Input: part model. Units: mm. Frame: model coordinates. A direction names the side the tool comes from. Coordinates: 2 decimals unless noted, no trailing zeros. Loops run counter-clockwise (first coordinate to the right, second up) from the corner with the lowest first, then second, coordinate; pieces in that order, holes last.
Item 1: Section D-D on z = -22.5. Return loops of the section in (x, y).
Item 2: Ray query, line 1 along X through (y, z) = (45.9, 2.9) (3 decimals); line 2 along Y through (x, z) = (-42.6, 3.95) (3 decimals); line 3 along Y through (x, z) = (59, 1.35) (3 decimals). Return the intervals inside material, ascending.
Item 3: Section C-C on x = -42.6. Return loops of the section in (y, z) (3 decimals), and give its area (3 significant figures).
Item 4: Contact query for flat-ended pins moving along their axis: P1, Ø8.5, axis at x = -42.6, y = 45.9, coming from the -Z side; P2, Ø5.5, axis at x = 8.2, y = -56.4, coming from the +Z side; P3, Ø6, axis at x = -43.5, z = -10.5, coming from the +Y side; P4, Ø3, axis at x = -50, z = -4.5, coming from the +Y side. Output: stop coordinate, or through.
Item 5: Reachability of faces 4 (the flat face through (-1, 3, 0)), 5 (the cylindrical face through (62.03, 46.85, 2.85)) from +Z, -Z, +X, -X, +Y, -Y: full face, straight path, thin tool, end or side. Return the list, or none.
Item 6: Section A-A on x = 77. Return loops of the section in (y, z).
Item 7: Section B-B on y = 45.9. Return loops of the section in (x, z) (3 decimals), and give its area (3 significant figures).
Item 8: Pull-direction query (Y, two-part tool) for faces 1 (the cylindrical face through (5.68, -58.33, 2.85)), 2 (the flat face through (1, -73.66, -7)), 3 (the flat face through (79, -77, -40.64)); classes: released by +Y, released by -Y, zero draft, split by the parting line, or undercut.
```python
from build123d import *

# Parameters (mm, degrees)
SKETCH1_W                  = 169
SKETCH1_H                  = 152.4
BOSS_EXTRUDE1_DEPTH        = 2.54
SKETCH2_W                  = 169
SKETCH2_H                  = 2.54
BOSS_EXTRUDE2_DEPTH        = 40.64
CUT_EXTRUDE1_REACH         = 122.823
SKETCH4_R                  = 3.175
CUT_EXTRUDE2_REACH         = 178.776
SKETCH3_R                  = 3.020871564
SKETCH3_R_2                = 97.5
CONVERT_SOLID1_START       = -5.790000104
CONVERT_SOLID1_OUTLINE_W   = 169
CONVERT_SOLID1_OUTLINE_H   = 149.86
CONVERT_SOLID1_OUTLINE_R   = 3.175
CONVERT_SOLID1_DEPTH       = 11.580006304
CONVERT_SOLID1_START_2     = -40.64
CONVERT_SOLID1_2_OUTLINE_W = 169
CONVERT_SOLID1_2_OUTLINE_H = 3.2500062
CONVERT_SOLID1_2_DEPTH     = 43.18
CONVERT_SOLID1_START_3     = 2.54
CONVERT_SOLID1_3_OUTLINE_W = 169
CONVERT_SOLID1_3_OUTLINE_H = 2.54
CONVERT_SOLID1_3_DEPTH     = 2.060276352
CONVERT_SOLID1_START_4     = -67.869999896
CONVERT_SOLID1_4_OUTLINE_W = 169
CONVERT_SOLID1_4_OUTLINE_H = 5.790000104
CONVERT_SOLID1_4_DEPTH     = 144.069999896
CONVERT_SOLID1_START_5     = -79.4500062
CONVERT_SOLID1_5_OUTLINE_R = 3.020871564
CONVERT_SOLID1_5_DEPTH     = 3.2500062
CONVERT_SOLID1_6_OUTLINE_W = 169
CONVERT_SOLID1_6_OUTLINE_H = 2.54
CONVERT_SOLID1_6_DEPTH     = 0.546460785
CONVERT_SOLID1_START_6     = -85
CONVERT_SOLID1_7_DEPTH     = 170


with BuildPart() as part:
    # Sketch1 → Boss-Extrude1 (new body)
    with BuildSketch(Plane.XY):
        Rectangle(SKETCH1_W, SKETCH1_H)
    extrude(amount=BOSS_EXTRUDE1_DEPTH)

    # Sketch2 → Boss-Extrude2 (add)
    with BuildSketch(Plane(origin=(0, 0, 0), x_dir=(-1, 0, 0), z_dir=(0, 0, -1))):
        with Locations((0, -74.93)):
            Rectangle(SKETCH2_W, SKETCH2_H)
    extrude(amount=BOSS_EXTRUDE2_DEPTH)

    # Sketch4 → Cut-Extrude1 (cut, up to next)
    with BuildSketch(Plane(origin=(0, 0, 0), x_dir=(-1, 0, 0), z_dir=(0, 0, -1)), mode=Mode.PRIVATE) as cut_extrude1_sk1:
        with Locations((-59, 45.9)):
            Circle(SKETCH4_R)
    cut_extrude1_tool1 = extrude(cut_extrude1_sk1.sketch, amount=-CUT_EXTRUDE1_REACH, mode=Mode.PRIVATE) & part.part
    # Sketch4 → Cut-Extrude1 (cut, up to next)
    with BuildSketch(Plane(origin=(0, 0, 0), x_dir=(-1, 0, 0), z_dir=(0, 0, -1)), mode=Mode.PRIVATE) as cut_extrude1_sk2:
        with Locations((-59, -56.4)):
            Circle(SKETCH4_R)
    cut_extrude1_tool2 = extrude(cut_extrude1_sk2.sketch, amount=-CUT_EXTRUDE1_REACH, mode=Mode.PRIVATE) & part.part
    # Sketch4 → Cut-Extrude1 (cut, up to next)
    with BuildSketch(Plane(origin=(0, 0, 0), x_dir=(-1, 0, 0), z_dir=(0, 0, -1)), mode=Mode.PRIVATE) as cut_extrude1_sk3:
        with Locations((-8.2, 45.9)):
            Circle(SKETCH4_R)
    cut_extrude1_tool3 = extrude(cut_extrude1_sk3.sketch, amount=-CUT_EXTRUDE1_REACH, mode=Mode.PRIVATE) & part.part
    # Sketch4 → Cut-Extrude1 (cut, up to next)
    with BuildSketch(Plane(origin=(0, 0, 0), x_dir=(-1, 0, 0), z_dir=(0, 0, -1)), mode=Mode.PRIVATE) as cut_extrude1_sk4:
        with Locations((42.6, 45.9)):
            Circle(SKETCH4_R)
    cut_extrude1_tool4 = extrude(cut_extrude1_sk4.sketch, amount=-CUT_EXTRUDE1_REACH, mode=Mode.PRIVATE) & part.part
    # Sketch4 → Cut-Extrude1 (cut, up to next)
    with BuildSketch(Plane(origin=(0, 0, 0), x_dir=(-1, 0, 0), z_dir=(0, 0, -1)), mode=Mode.PRIVATE) as cut_extrude1_sk5:
        with Locations((42.6, -56.4)):
            Circle(SKETCH4_R)
    cut_extrude1_tool5 = extrude(cut_extrude1_sk5.sketch, amount=-CUT_EXTRUDE1_REACH, mode=Mode.PRIVATE) & part.part
    # Sketch4 → Cut-Extrude1 (cut, up to next)
    with BuildSketch(Plane(origin=(0, 0, 0), x_dir=(-1, 0, 0), z_dir=(0, 0, -1)), mode=Mode.PRIVATE) as cut_extrude1_sk6:
        with Locations((-8.2, -56.4)):
            Circle(SKETCH4_R)
    cut_extrude1_tool6 = extrude(cut_extrude1_sk6.sketch, amount=-CUT_EXTRUDE1_REACH, mode=Mode.PRIVATE) & part.part
    add(cut_extrude1_tool1.solids().sort_by_distance((59, 45.9, 0))[0], mode=Mode.SUBTRACT)
    add(cut_extrude1_tool2.solids().sort_by_distance((59, -56.4, 0))[0], mode=Mode.SUBTRACT)
    add(cut_extrude1_tool3.solids().sort_by_distance((8.2, 45.9, 0))[0], mode=Mode.SUBTRACT)
    add(cut_extrude1_tool4.solids().sort_by_distance((-42.6, 45.9, 0))[0], mode=Mode.SUBTRACT)
    add(cut_extrude1_tool5.solids().sort_by_distance((-42.6, -56.4, 0))[0], mode=Mode.SUBTRACT)
    add(cut_extrude1_tool6.solids().sort_by_distance((8.2, -56.4, 0))[0], mode=Mode.SUBTRACT)

    # Sketch3 → Cut-Extrude2 (cut, up to next)
    with BuildSketch(Plane(origin=(0, -73.66, 0), x_dir=(1, 0, 0), z_dir=(0, 1, 0)), mode=Mode.PRIVATE) as cut_extrude2_sk1:
        with Locations(Location((77, 28.473587136, 0), (0, 0, 180))):
            Circle(SKETCH3_R)
    cut_extrude2_tool1 = extrude(cut_extrude2_sk1.sketch, amount=-CUT_EXTRUDE2_REACH, mode=Mode.PRIVATE) & part.part
    # Sketch3 → Cut-Extrude2 (cut, up to next)
    with BuildSketch(Plane(origin=(0, -73.66, 0), x_dir=(1, 0, 0), z_dir=(0, 1, 0)), mode=Mode.PRIVATE) as cut_extrude2_sk2:
        with Locations(Location((-77, 28.473587136, 0), (0, 0, 180))):
            Circle(SKETCH3_R)
    cut_extrude2_tool2 = extrude(cut_extrude2_sk2.sketch, amount=-CUT_EXTRUDE2_REACH, mode=Mode.PRIVATE) & part.part
    # Sketch3 → Cut-Extrude2 (cut, up to next)
    with BuildSketch(Plane(origin=(0, -73.66, 0), x_dir=(1, 0, 0), z_dir=(0, 1, 0)), mode=Mode.PRIVATE) as cut_extrude2_sk3:
        with Locations((0, 105.473587136)):
            Circle(SKETCH3_R_2)
    cut_extrude2_tool3 = extrude(cut_extrude2_sk3.sketch, amount=-CUT_EXTRUDE2_REACH, mode=Mode.PRIVATE) & part.part
    add(cut_extrude2_tool1.solids().sort_by_distance((77, -73.66, -28.473587))[0], mode=Mode.SUBTRACT)
    add(cut_extrude2_tool2.solids().sort_by_distance((-77, -73.66, -28.473587))[0], mode=Mode.SUBTRACT)
    add(cut_extrude2_tool3.solids().sort_by_distance((0, -73.66, -105.473587))[0], mode=Mode.SUBTRACT)

    # Convert-Solid1: read off the stored shape, not the designer's step
    # Convert-Solid1 outline → Convert-Solid1 (add)
    with BuildSketch(Plane.XY.offset(CONVERT_SOLID1_START)):
        with Locations((0, 1.27)):
            Rectangle(CONVERT_SOLID1_OUTLINE_W, CONVERT_SOLID1_OUTLINE_H)
        with Locations((-42.6, -56.4)):
            Circle(CONVERT_SOLID1_OUTLINE_R, mode=Mode.SUBTRACT)
        with Locations((8.2, -56.4)):
            Circle(CONVERT_SOLID1_OUTLINE_R, mode=Mode.SUBTRACT)
        with Locations((59, -56.4)):
            Circle(CONVERT_SOLID1_OUTLINE_R, mode=Mode.SUBTRACT)
        with Locations((-42.6, 45.9)):
            Circle(CONVERT_SOLID1_OUTLINE_R, mode=Mode.SUBTRACT)
        with Locations((8.2, 45.9)):
            Circle(CONVERT_SOLID1_OUTLINE_R, mode=Mode.SUBTRACT)
        with Locations((59, 45.9)):
            Circle(CONVERT_SOLID1_OUTLINE_R, mode=Mode.SUBTRACT)
    extrude(amount=CONVERT_SOLID1_DEPTH)

    # Convert-Solid1 2 outline → Convert-Solid1 2 (add)
    with BuildSketch(Plane.XY.offset(CONVERT_SOLID1_START_2)):
        with Locations((0, -77.8250031)):
            Rectangle(CONVERT_SOLID1_2_OUTLINE_W, CONVERT_SOLID1_2_OUTLINE_H)
    extrude(amount=CONVERT_SOLID1_2_DEPTH)

    # Convert-Solid1 3 outline → Convert-Solid1 3 (add)
    with BuildSketch(Plane.XY.offset(CONVERT_SOLID1_START_3)):
        with Locations((0, -74.93)):
            Rectangle(CONVERT_SOLID1_3_OUTLINE_W, CONVERT_SOLID1_3_OUTLINE_H)
    extrude(amount=CONVERT_SOLID1_3_DEPTH)

    # Convert-Solid1 4 outline → Convert-Solid1 4 (cut)
    with BuildSketch(Plane(origin=(0, 0, 0), x_dir=(1, 0, 0), z_dir=(0, 1, 0)).offset(CONVERT_SOLID1_START_4)):
        with Locations((0, 2.895000052)):
            Rectangle(CONVERT_SOLID1_4_OUTLINE_W, CONVERT_SOLID1_4_OUTLINE_H)
    extrude(amount=CONVERT_SOLID1_4_DEPTH, mode=Mode.SUBTRACT)

    # Convert-Solid1 5 outline → Convert-Solid1 5 (cut)
    with BuildSketch(Plane(origin=(0, 0, 0), x_dir=(1, 0, 0), z_dir=(0, 1, 0)).offset(CONVERT_SOLID1_START_5)):
        with BuildLine():
            Line((72.820711196, 40.64), (-72.820711196, 40.64))
            ThreePointArc((-72.820711196, 40.64), (0, 7.973587136), (72.820711196, 40.64))
        make_face()
        with Locations((-77, 28.473587136)):
            Circle(CONVERT_SOLID1_5_OUTLINE_R)
        with Locations((77, 28.473587136)):
            Circle(CONVERT_SOLID1_5_OUTLINE_R)
    extrude(amount=CONVERT_SOLID1_5_DEPTH, mode=Mode.SUBTRACT)

    # Convert-Solid1 6 outline → Convert-Solid1 6 (cut)
    with BuildSketch(Plane(origin=(0, 0, 0), x_dir=(1, 0, 0), z_dir=(0, 1, 0)).offset(CONVERT_SOLID1_START_5)):
        with Locations((0, -1.27)):
            Rectangle(CONVERT_SOLID1_6_OUTLINE_W, CONVERT_SOLID1_6_OUTLINE_H)
    extrude(amount=CONVERT_SOLID1_6_DEPTH, mode=Mode.SUBTRACT)

    # Convert-Solid1 7 outline → Convert-Solid1 7 (cut)
    with BuildSketch(Plane.YZ.offset(CONVERT_SOLID1_START_6)):
        with BuildLine():
            Line((-67.869999896, -5.790000104), (-67.869999896, 0))
            ThreePointArc((-67.869999896, 0), (-71.964148233, -1.695851767), (-73.66, -5.790000104))
            Line((-73.66, -5.790000104), (-67.869999896, -5.790000104))
        make_face()
        with BuildLine():
            ThreePointArc((-79.4500062, -5.790000104), (-76.05830088, 2.39830088), (-67.869999896, 5.7900062))
            Line((-67.869999896, 5.7900062), (-73.66, 5.7900062))
            Line((-73.66, 5.7900062), (-73.66, 4.600276352))
            Line((-73.66, 4.600276352), (-76.2, 4.600276352))
            Line((-76.2, 4.600276352), (-76.2, 2.54))
            Line((-76.2, 2.54), (-78.903545415, 2.54))
            Line((-78.903545415, 2.54), (-78.903545415, 0))
            Line((-78.903545415, 0), (-79.4500062, 0))
            Line((-79.4500062, 0), (-79.4500062, -5.790000104))
        make_face()
    extrude(amount=CONVERT_SOLID1_7_DEPTH, mode=Mode.SUBTRACT)


solid = part.part
```
Results found:
1. outline: (-84.5, -79.45) - (-51.2, -79.45) - (-51.2, -73.66) - (-84.5, -73.66) - close; (51.2, -79.45) - (84.5, -79.45) - (84.5, -73.66) - (51.2, -73.66) - close
2. line 1: x = -84.5 to -45.775, -39.425 to 5.025, 11.375 to 55.825, 62.175 to 84.5
2. line 2: y = -74.133 to -59.575, -53.225 to 42.725, 49.075 to 76.2
2. line 3: y = -76.987 to -59.575, -53.225 to 42.725, 49.075 to 76.2
3. outline: (-79.45, -17.772) - (-73.66, -17.772) - (-73.66, -5.79) arc R5.79 cw to (-67.87, 0) - (-59.575, 0) - (-59.575, 5.79) - (-67.87, 5.79) arc R11.58 ccw to (-79.45, -5.79) - close; (-53.225, 0) - (42.725, 0) - (42.725, 5.79) - (-53.225, 5.79) - close; (49.075, 0) - (76.2, 0) - (76.2, 5.79) - (49.075, 5.79) - close
3. area: 909 mm2
4. P1: stops at z = 0
4. P2: passes through
4. P3: stops at y = -73.66
4. P4: stops at y = -72.94
5. face 4: -Z, +X, -X, +Y
5. face 5: +Z, -Z
6. outline: (-79.45, -40.64) - (-73.66, -40.64) - (-73.66, -31.49) - (-79.45, -31.49) - close; (-79.45, -25.45) - (-73.66, -25.45) - (-73.66, -5.79) arc R5.79 cw to (-67.87, 0) - (76.2, 0) - (76.2, 5.79) - (-67.87, 5.79) arc R11.58 ccw to (-79.45, -5.79) - close
7. outline: (-84.5, 0) - (-45.775, 0) - (-45.775, 5.79) - (-84.5, 5.79) - close; (-39.425, 0) - (5.025, 0) - (5.025, 5.79) - (-39.425, 5.79) - close; (11.375, 0) - (55.825, 0) - (55.825, 5.79) - (11.375, 5.79) - close; (62.175, 0) - (84.5, 0) - (84.5, 5.79) - (62.175, 5.79) - close
7. area: 868 mm2
8. face 1: undercut
8. face 2: released by +Y
8. face 3: zero draft
